CAD build for the part. Positions are in the model's coordinates, mm. A direction names the side the tool comes from. Coordinates: 2 decimals unless noted, no trailing zeros. Loops run counter-clockwise (first coordinate to the right, second up) from the corner with the lowest first, then second, coordinate; pieces in that order, holes last.
1) Saw through at C-C, the plane z = -3. Write the cut outline in (x, y), and give its area (3 significant figures).
2) Saw through at B-B, the plane y = 0. Give the number of separate pieces and of enclosed holes in the cut face, and give its area (3 significant figures).
3) Pin check, flat tips, straight feed: pin 1 Ø8.5 at (y, z) = (0, -14.015) entering from -X; pin 2 Ø7 at (x, y) = (-12, 20.78) entering from -Z; pin 3 Ø5.5 at (x, y) = (12, -20.78) entering from -Z; pin 4 Ø5 at (y, z) = (18, -6) entering from +X. Stop position of each tip, or through.
4) Which spindle directions (+Z, -Z, +X, -X, +Y, -Y) get a long thin tool onto all of the face, cutting with end or side? Do faces 4 (the cylindrical face through (-13.411, 0.413, -17.163)), 5 (the flat face through (-19, 0, 8)), 6 (the flat face through (-19, 0, 0)), 7 (the flat face through (2.55, -11, -5)). Say none if no direction does.
5) Wall check: line 1 along Z through (x, y) = (-13, 0); line 2 along X through (y, z) = (0, -7); line 3 along Z through (x, y) = (-25.5, 9.5). Give the ranges that are in metal, low to high.
6) Two-plate mould, pull along Y, no slides. Class faces 1 (the cylindrical face through (14.211, 22.812, 3.944)), 2 (the flat face through (-7.2, 7.2, 11)), 3 (the cylindrical face through (-18.06, -4.01, -3.47)): +Y half, -Y half, draft (parallel to the pull), parting line (faces both ways), or undercut.
7) Saw through at D-D, the plane x = 24. Write the cut outline in (y, z).
8) Saw through at A-A, the plane z = 3.5. Write the cut outline in (x, y).
```python
from build123d import *

# Parameters (mm, degrees)
CUT_EXTRUDE1_DEPTH      = 12
CUT_EXTRUDE1_DEPTH_BACK = 22
SKETCH3_R               = 3
CUT_EXTRUDE2_DEPTH      = 22
CUT_EXTRUDE2_DEPTH_BACK = 12
SKETCH4_R               = 3.175
CUT_EXTRUDE3_DEPTH      = 30
CUT_EXTRUDE3_DEPTH_BACK = 30


with BuildPart() as part:
    # Sketch1 → Revolve1 (revolve)
    with BuildSketch(Plane(origin=(0, 0, 0), x_dir=(0, 0, -1), z_dir=(1, 0, 0))):
        Polygon((21, 17.45), (7.03, 17.45), (7.03, 18.5), (0, 18.5), (0, 29), (-8, 29), (-8, 18.586235054), (-11, 16.803216346), (-11, 10), (21, 10), align=None)
    revolve(axis=Axis((0, 0, 11), (0, 0, -1)))

    # Sketch2 → Cut-Extrude1 (cut, two sides)
    with BuildSketch(Plane.XY) as cut_extrude1_sk:
        with BuildLine():
            Line((-2.55, -12.75), (2.55, -12.75))
            Line((2.55, -12.75), (2.55, -9.66941053))
            ThreePointArc((2.55, -9.66941053), (0, -10), (-2.55, -9.66941053))
            Line((-2.55, -9.66941053), (-2.55, -12.75))
        make_face()
    extrude(amount=CUT_EXTRUDE1_DEPTH, mode=Mode.SUBTRACT)
    extrude(cut_extrude1_sk.sketch, amount=-CUT_EXTRUDE1_DEPTH_BACK, mode=Mode.SUBTRACT)

    # Sketch3 → Cut-Extrude2 (cut, two sides)
    with BuildSketch(Plane(origin=(0, 0, 0), x_dir=(-1, 0, 0), z_dir=(0, 0, -1))) as cut_extrude2_sk:
        with Locations((-24, 0)):
            Circle(SKETCH3_R)
        with Locations((-12, 20.784609691)):
            Circle(SKETCH3_R)
        with Locations((12, 20.784609691)):
            Circle(SKETCH3_R)
        with Locations((24, 0)):
            Circle(SKETCH3_R)
        with Locations((12, -20.784609691)):
            Circle(SKETCH3_R)
        with Locations((-12, -20.784609691)):
            Circle(SKETCH3_R)
    extrude(amount=CUT_EXTRUDE2_DEPTH, mode=Mode.SUBTRACT)
    extrude(cut_extrude2_sk.sketch, amount=-CUT_EXTRUDE2_DEPTH_BACK, mode=Mode.SUBTRACT)

    # Sketch4 → Cut-Extrude3 (cut, two sides)
    with BuildSketch(Plane(origin=(0, 0, 0), x_dir=(0, -1, 0), z_dir=(1, 0, 0))) as cut_extrude3_sk:
        with Locations((0, 14.015)):
            Circle(SKETCH4_R)
    extrude(amount=CUT_EXTRUDE3_DEPTH, mode=Mode.SUBTRACT)
    extrude(cut_extrude3_sk.sketch, amount=-CUT_EXTRUDE3_DEPTH_BACK, mode=Mode.SUBTRACT)


solid = part.part
```
Data:
1. outline: circle Ø37 at (0, 0); hole (-2.55, -12.75) - (2.55, -12.75) - (2.55, -9.67) arc R10 ccw (long way) to (-2.55, -9.67) - close
1. area: 746 mm2
2. separate pieces: 6
2. enclosed holes: 0
2. area: 487 mm2
3. pin 1: stops at x = -17.45
3. pin 2: stops at z = 0
3. pin 3: passes through
3. pin 4: stops at x = 10.1
4. face 4: +X, -X
4. face 5: +Z
4. face 6: -Z
4. face 7: +Z, -Z
5. line 1: z = -21 to -17.19, -10.84 to 11
5. line 2: x = -18.5 to -10, 10 to 18.5
5. line 3: z = 0 to 8
6. face 1: undercut
6. face 2: draft
6. face 3: parting line
7. outline: (-16.28, 0) - (-3, 0) - (-3, 8) - (-16.28, 8) - close; (3, 0) - (16.28, 0) - (16.28, 8) - (3, 8) - close
8. outline: circle Ø58 at (0, 0); hole circle Ø6 at (-24, 0); hole circle Ø6 at (-12, -20.78); hole circle Ø6 at (-12, 20.78); hole (-2.55, -12.75) - (2.55, -12.75) - (2.55, -9.67) arc R10 ccw (long way) to (-2.55, -9.67) - close; hole circle Ø6 at (12, -20.78); hole circle Ø6 at (12, 20.78); hole circle Ø6 at (24, 0)
